The listing builds one solid part. Answer for the finished solid, in the listing's coordinates (mm). A direction names the side the tool comes from. Give positions to 0.01 mm unless a question says otherwise; leave off trailing zeros. Order: outer loops, then holes, each group sorted by start corner. A loop starts at its lowest first (then second) coordinate and runs counter-clockwise, first axis right, second up.
Autodesk Inventor part; units mm, degrees
ref_plane "YZ Plane" through (0, 0, 0) normal (1, 0, 0) x (0, 1, 0)
ref_plane "XZ Plane" through (0, 0, 0) normal (0, 1, 0) x (-1, 0, 0)
ref_plane "XY Plane" through (0, 0, 0) normal (0, 0, 1) x (1, 0, 0)
sketch "Sketch1" plane through (0, 0, 0) normal (0, 1, 0) x (-1, 0, 0)
  circle A0 centre (0, 0) radius 6.5
  line L0 (0, 6.5) -> (15, 6.5)
  line L1 (15, 6.5) -> (15, -6.5)
  line L2 (15, -6.5) -> (0, -6.5)
  line L3 (0, -6.5) -> (0, 6.5)
  line L4 (15, 2.5) -> (85, 2.5)
  line L5 (85, 2.5) -> (85, -2.5)
  line L6 (85, -2.5) -> (15, -2.5)
  line L7 (15, -2.5) -> (15, 2.5)
  dimension "d0" = 13
  dimension "d1" = 6.5
  dimension "d2" = 15
  dimension "d3" = 6.5
  dimension "d4" = 70
  dimension "d5" = 4
  dimension "d6" = 4
extrude "Extrusion1" add sketch "Sketch1" along normal blind 4
fillet "Fillet1" radius 2 2 edges at (-50, 4, -2.5) (-50, 0, -2.5)
properties part number "Arms"
1) Find section B-B (y = 0.65). Write down the section's boundary in (x, z), then the cut area to 3 significant figures.
Geometry says:
outline: (-85, -1.98) - (-15, -1.98) - (-15, -6.5) - (0, -6.5) arc R6.5 ccw to (0, 6.5) - (-15, 6.5) - (-15, 2.5) - (-85, 2.5) - close
area: 575 mm2
2) Straight lines are drawn through the part: probe 1 along Z at (x, y) = (-20.5, 2.25); probe 2 along X at (y, z) = (2.2, -0.5); probe 3 along X at (y, z) = (0.2, -1.75). For each, find the intervals that lie inside material, in ascending order.
Geometry says:
probe 1: z = -2.48 to 2.5
probe 2: x = -85 to 6.48
probe 3: x = -15 to 6.26
3) Find section D-D (z = -3.75). Write down the section's boundary in (x, y).
Geometry says:
outline: (-15, 0) - (5.31, 0) - (5.31, 4) - (-15, 4) - close
4) A tool of negligible diameter and unlimited length cuts with its end or side. For faces 1 (the flat face through (-8, 2, -6.5)), 2 (the cylindrical face through (-49.51, 0.57, -1.9)), 3 (the cylindrical face through (-49.51, 3.4, -1.93)), 4 (the flat face through (-50, 2, 2.5)), from which of +Z, -Z, +X, -X, +Y, -Y can it reach the whole face along a straight path? Write none if from no direction.
Geometry says:
face 1: -Z, +X, -X, +Y, -Y
face 2: -Z, -X, -Y
face 3: -Z, -X, +Y
face 4: +Z, -X, +Y, -Y
5) Given P1, Ø1.5, axis at x = -63, y = 1, coming from the -Z side; P2, Ø1, axis at x = -18, z = -2.5, coming from the -Y side; P3, Ø2, axis at x = -41, y = 1.5, coming from the +Z side, each flat-ended and moving along its own axis, determine where each tip first touches the part or whether it passes through.
Geometry says:
P1: stops at z = -2.48
P2: stops at y = 0.68
P3: stops at z = 2.5
6) Find section C-C (z = 4.25). Write down the section's boundary in (x, y).
Geometry says:
outline: (-15, 0) - (4.92, 0) - (4.92, 4) - (-15, 4) - close
